Work out the finished part from the listing and answer in its coordinate system (mm). Face numbers are marked on the shaded views. A direction names the side the tool comes from. Give positions to 0.01 mm unless a question says otherwise; leave off trailing zeros. Order: outer loops, then holes, each group sorted by start corner. A loop starts at its lowest first (then second) coordinate and runs counter-clockwise, first axis right, second up. Notation, with made-up numbers: (-8.75, 22) - (45.25, 22) arc R21 cw to (45.25, 43) - close; hole circle Ø4 at (-12, 2.5). An arc over 180 degrees is marked (long way). Put each result on its own line as item: value.
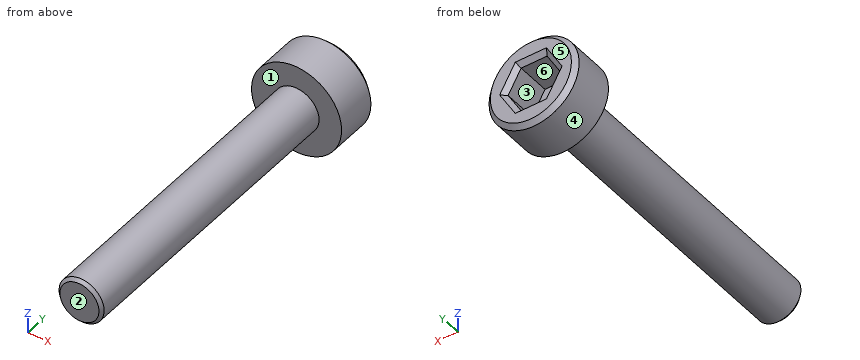
```python
from build123d import *

# Parameters (mm, degrees)
SKETCH1_R           = 3
BOSS_EXTRUDE1_DEPTH = 3
CHAMFER1_SIZE       = 0.3
CUT_EXTRUDE1_DEPTH  = 2.5
CHAMFER2_SIZE       = 0.3
SKETCH3_R           = 1.5
BOSS_EXTRUDE2_DEPTH = 20
CHAMFER3_SIZE       = 0.2


with BuildPart() as part:
    # Sketch1 → Boss-Extrude1 (new body)
    with BuildSketch(Plane(origin=(0, 0, 0), x_dir=(1, 0, 0), z_dir=(0, 1, 0))):
        with Locations(Location((0, 0, 0), (0, 0, 270))):  # turned: the seam where the file's is
            Circle(SKETCH1_R)
    extrude(amount=BOSS_EXTRUDE1_DEPTH)

    # Chamfer1
    chamfer1_edges = [part.edges().sort_by_distance(p)[0] for p in [
        (0, 3, -3),
    ]]
    chamfer(chamfer1_edges, length=CHAMFER1_SIZE)

    # Sketch2 → Cut-Extrude1 (cut)
    with BuildSketch(Plane(origin=(0, 3, 0), x_dir=(1, 0, 0), z_dir=(0, 1, 0))):
        Polygon((1.732050808, 0), (0.866025404, 1.5), (-0.866025404, 1.5), (-1.732050808, 0), (-0.866025404, -1.5), (0.866025404, -1.5), align=None)
    extrude(amount=-CUT_EXTRUDE1_DEPTH, mode=Mode.SUBTRACT)

    # Chamfer2
    chamfer2_edges = [part.edges().sort_by_distance(p)[0] for p in [
        (1.299038106, 3, 0.75),
        (1.299038106, 3, -0.75),
        (0, 3, -1.5),
        (-1.299038106, 3, -0.75),
        (-1.299038106, 3, 0.75),
        (0, 3, 1.5),
    ]]
    chamfer(chamfer2_edges, length=CHAMFER2_SIZE)

    # Sketch3 → Boss-Extrude2 (add)
    with BuildSketch(Plane.XZ):
        with Locations(Location((0, 0, 0), (0, 0, 90))):  # turned: the seam where the file's is
            Circle(SKETCH3_R)
    extrude(amount=BOSS_EXTRUDE2_DEPTH)

    # Chamfer3
    chamfer3_edges = [part.edges().sort_by_distance(p)[0] for p in [
        (0, -20, -1.5),
    ]]
    chamfer(chamfer3_edges, length=CHAMFER3_SIZE)


solid = part.part
```
(1) Given pin 1 (1.5 mm diameter, centred on x = -1.5, z = 1.5, fed in from -Y), flat-ended and moving along its own axis, determine where the tip first touches the part or whether it passes through.
Geometry check:
pin 1: stops at y = -19.93
(2) Straight lines are drawn through the part: line 1 (Y direction, x = -0.25, z = 2.25); line 2 (X direction, y = -12.5, z = -0.1); line 3 (Z direction, x = 1, y = 1.5). For each, find the intervals that lie inside material, in ascending order.
Geometry check:
line 1: y = 0 to 3
line 2: x = -1.5 to 1.5
line 3: z = -2.83 to -1.27, 1.27 to 2.83
(3) A tool of negligible diameter and unlimited length cuts with its end or side. For the marked faces 1, 2 and 3, from which of +Z, -Z, +X, -X, +Y, -Y can it reach the whole face along a straight path? Write none if from no direction.
Geometry check:
face 1: -Y
face 2: +Z, -Z, +X, -X, -Y
face 3: +Y
(4) Section C-C, the plane y = -11.5 is taken. Write down the section's boundary in (x, z).
Geometry check:
outline: circle Ø3 at (0, 0)
(5) Section B-B, the plane x = 0 is taken. Write down the section's boundary in (y, z), then the cut area to 3 significant figures.
Geometry check:
outline: (-20, -1.3) - (-19.8, -1.5) - (0, -1.5) - (0, -3) - (2.7, -3) - (3, -2.7) - (3, -1.8) - (2.7, -1.5) - (0.5, -1.5) - (0.5, 1.5) - (2.7, 1.5) - (3, 1.8) - (3, 2.7) - (2.7, 3) - (0, 3) - (0, 1.5) - (-19.8, 1.5) - (-20, 1.3) - close
area: 70.3 mm²
(6) Determine the mould class of the marked faces 4, 5 and 6 for opening direction Z: pulls with the +Z half, pulls with the -Z half, needs draft (parallel to the pull), parting line crosses it, or undercut.
Geometry check:
face 4: parting line crosses it
face 5: needs draft
face 6: undercut
(7) Section A-A, the plane y = 1.25 is taken. Write down the section's boundary in (x, z), then the cut area to 3 significant figures.
Geometry check:
outline: circle Ø6 at (0, 0); hole (-1.73, 0) - (-0.87, -1.5) - (0.87, -1.5) - (1.73, 0) - (0.87, 1.5) - (-0.87, 1.5) - close
area: 20.5 mm²
